Job drawing, mm, ordinate dimensions from the low corner. One solid piece. A direction names the side the tool comes from. Give positions to 0.01 mm unless a question says otherwise; leave off trailing zeros. Order: outer loops, then holes, each group sorted by start corner. A loop starts at its lowest first (then second) coordinate and runs counter-clockwise, first axis right, second up. Notation, with made-up numbers: M 86.5,56 L 107.5,56 A19 ccw 107.5,82 Z; hole C -2,-20.75 d6. An arc over 180 degrees is marked long. One line per question, with ' | ' between items.
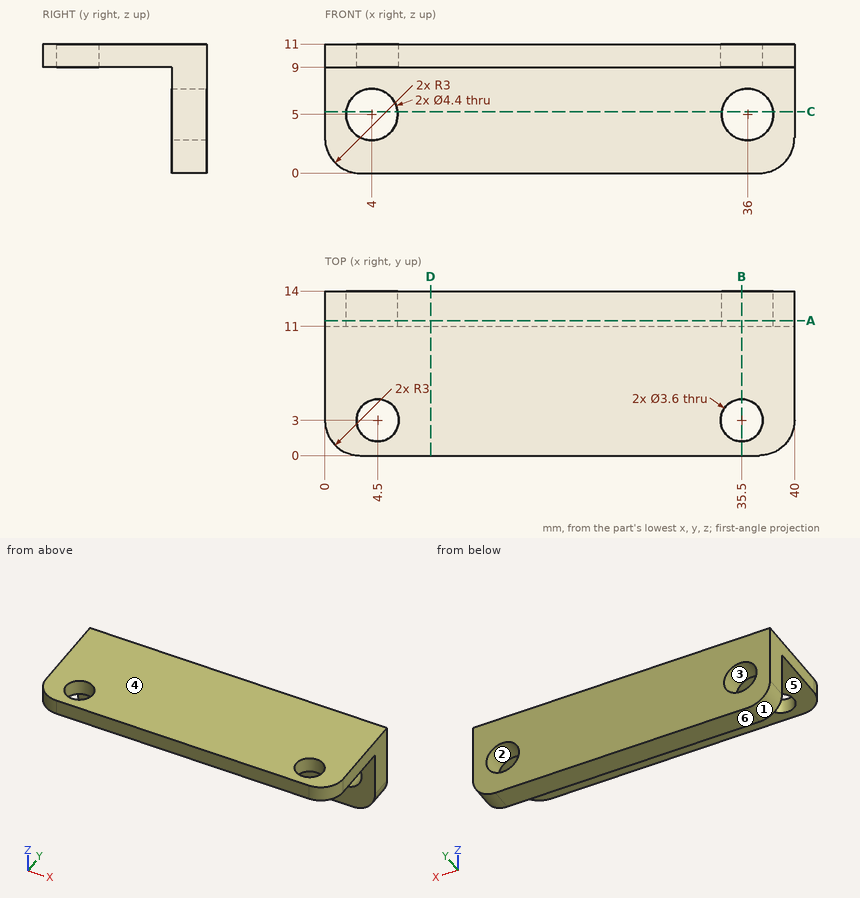
1. Slice it at A-A on y = 11.5. Give the cut face in (x, z).
Worked out:
outline: M 0,3 A3 ccw 3,0 L 37,0 A3 ccw 40,3 L 40,11 L 0,11 Z; hole C 4,5 d4.4; hole C 36,5 d4.4
2. Tool access for the marked faces 5 and 6: list every direction of +Z, -Z, +X, -X, +Y, -Y with a clear straight run to the whole face (end or side of a thin tool).
Worked out:
face 5: -Z, +X, -X, -Y | face 6: -Z, +X, -X, +Y, -Y
3. Probe L1, parallel to X at y = 13.05, z = 5; L2, parallel to Z at x = 4, y = 12.85; L3, parallel to Y at x = 4.5, z = 10.05. List the from-to ranges inside material, lowest first. Write a range as from..to.
Worked out:
L1: x = 0..1.8, 6.2..33.8, 38.2..40 | L2: z = 0..2.8, 7.2..11 | L3: y = 0..1.2, 4.8..14
4. Drop flat-ended pins along their axis: pin 1 (4.5 mm diameter, centred on x = 15.5, z = 6, fed in from -Y); pin 2 (5.5 mm diameter, centred on x = 16.5, y = 4.5, fed in from -Z). Give the stop position or say it passes through.
Worked out:
pin 1: stops at y = 11 | pin 2: stops at z = 9
5. Slice it at D-D on x = 9. Give the cut face in (y, z).
Worked out:
outline: M 0,9 L 11,9 L 11,0 L 14,0 L 14,11 L 0,11 Z
6. Slice it at C-C on z = 5.25. Give the cut face in (x, y), then the cut area to 3 significant figures.
Worked out:
outline: M 0,11 L 1.81,11 L 1.81,14 L 0,14 Z; M 6.19,11 L 33.81,11 L 33.81,14 L 6.19,14 Z; M 38.19,11 L 40,11 L 40,14 L 38.19,14 Z | area: 93.8 mm2
7. Mould opens along Z. For the marked faces 1, 2, 3 and 4 say: released by +Z, released by -Z, zero draft, split by the parting line, or undercut.
Worked out:
face 1: released by -Z | face 2: undercut | face 3: undercut | face 4: released by +Z
8. Slice it at B-B on x = 35.5. Give the cut face in (y, z), then the cut area to 3 significant figures.
Worked out:
outline: M 0,9 L 1.2,9 L 1.2,11 L 0,11 Z; M 4.8,9 L 11,9 L 11,7.14 L 14,7.14 L 14,11 L 4.8,11 Z; M 11,0 L 14,0 L 14,2.86 L 11,2.86 Z | area: 34.9 mm2
